from build123d import *

# Parameters (mm, degrees)
SKETCH1_R           = 34.925
BOSS_EXTRUDE1_DEPTH = 146.05
BOSS_EXTRUDE2_DEPTH = 3.175
LPATTERN1_COUNT     = 2
LPATTERN1_PITCH     = 149.225
SKETCH4_R           = 22.225
BOSS_EXTRUDE3_DEPTH = 25.4
SKETCH5_W           = 63.5
SKETCH5_H           = 63.5
BOSS_EXTRUDE4_DEPTH = 50.8
SKETCH6_R           = 9.525
BOSS_EXTRUDE5_DEPTH = 76.2


with BuildPart() as part:
    # Sketch1 → Boss-Extrude1 (new body)
    with BuildSketch(Plane.XY):
        Circle(SKETCH1_R)
    extrude(amount=BOSS_EXTRUDE1_DEPTH)

    # Sketch2 → Boss-Extrude2 (add)
    with BuildSketch(Plane.XY.offset(146.05)):
        Polygon((0, 0), (-38.1, -38.1), (38.1, -38.1), align=None)
    boss_extrude2 = extrude(amount=BOSS_EXTRUDE2_DEPTH)

    # LPattern1: Boss-Extrude2 ×2
    with Locations(*[(0, 0, -i * LPATTERN1_PITCH) for i in range(1, LPATTERN1_COUNT)]):
        add(boss_extrude2)

    # Sketch4 → Boss-Extrude3 (add)
    with BuildSketch(Plane.XY.offset(146.05)):
        with Locations(Location((0, 0, 0), (0, 0, 225))):
            Circle(SKETCH4_R)
    extrude(amount=BOSS_EXTRUDE3_DEPTH)

    # Sketch5 → Boss-Extrude4 (add)
    with BuildSketch(Plane(origin=(0, 33.02, 0), x_dir=(1, 0, 0), z_dir=(0, 1, 0))):
        with Locations((0, -127)):
            Rectangle(SKETCH5_W, SKETCH5_H)
    extrude(amount=BOSS_EXTRUDE4_DEPTH)

    # Sketch6 → Boss-Extrude5 (add)
    with BuildSketch(Plane(origin=(0, 0, 95.25), x_dir=(-1, 0, 0), z_dir=(0, 0, -1))):
        with Locations(Location((0, 74.295, 0), (0, 0, 90))):
            Circle(SKETCH6_R)
    extrude(amount=BOSS_EXTRUDE5_DEPTH)


solid = part.part
Input: part model. Units: mm. Frame: model coordinates. A direction names the side the tool comes from. Round coordinates to 2 decimals unless told otherwise and drop trailing zeros. Loops run counter-clockwise (first coordinate to the right, second up) from the corner with the lowest first, then second, coordinate; pieces in that order, holes last. Notation, with made-up numbers: M 15,11.5 L 57,11.5 A23 cw 57,39.5 Z; hole C 51,19 d9. An arc over 180 degrees is marked long. Answer as CSV lines item,"result". Start each with the question number.
(1) Line query: line 1 (Y direction, x = 0, z = 117) (3 decimals); line 2 (X direction, y = 34, z = 151.5); line 3 (X direction, y = -1.5, z = 60.5). Output: solid intervals per line, ascending. Write a range as [from, to].
(2) First-contact query: pin 1 (1.5 mm diameter, centred on x = 26, y = -22.5, fed in from -Z); pin 2 (15 mm diameter, centred on x = -11, y = 47.5, fed in from +Z); pin 3 (2 mm diameter, centred on x = -24, z = 67.5, fed in from -Y). Flat tips, straight axial feed; report the tip coordinate or a pass-through.
(3) Section D-D, the plane z = 102. Output: boundary loops of the cut face in (x, y) (3 decimals).
(4) Section C-C, the plane z = 45.5. Output: boundary loops of the cut face in (x, y) (3 decimals), plus the area to 3 significant figures.
(5) Section A-A, the plane x = 28. Output: boundary loops of the cut face in (y, z) (3 decimals).
(6) Reachability of faces 5 (the flat face through (31.75, 58, 127)), 6 (the flat face through (0, 74, 19.05)), 7 (the flat face through (27, -27, 148)) from +Z, -Z, +X, -X, +Y, -Y: full face, straight path, thin tool, end or side. Return the list, or none.
(7) Section B-B, the plane y = 49. Output: boundary loops of the cut face in (x, z).
(8) Draft query along Z for faces 1 (the flat face through (-1, -36, 146.05)), 2 (the flat face through (0, 58, 95.25)), 3 (the flat face through (-1, -36, 0)), 4 (the flat face through (19, -19, -2)). Return one class per face: released by +Z, released by -Z, zero draft, split by the parting line, or undercut.
Values found:
1,line 1,"y = [-34.925, 83.82]"
1,line 2,"x = [-31.75, 31.75]"
1,line 3,"x = [-34.89, 34.89]"
2,pin 1,"stops at z = 0"
2,pin 2,"stops at z = 158.75"
2,pin 3,"stops at y = -26.28"
3,outline,"M -31.75,33.02 L -11.377,33.02 A34.925 ccw long 11.377,33.02 L 31.75,33.02 L 31.75,83.82 L -31.75,83.82 Z"
4,outline,"C 0,0 d69.85; C 0,74.295 d19.05"
4,area,"4,120 mm²"
5,outline,"M -38.1,-3.175 L -28,-3.175 L -28,0 L -38.1,0 Z; M -38.1,146.05 L -28,146.05 L -28,149.225 L -38.1,149.225 Z; M -20.875,0 L 20.875,0 L 20.875,146.05 L -20.875,146.05 Z; M 33.02,95.25 L 83.82,95.25 L 83.82,158.75 L 33.02,158.75 Z"
6,face 5,"+Z, -Z, +X, +Y"
6,face 6,"-Z, +X, -X, +Y"
6,face 7,"+Z, +X"
7,outline,"M -31.75,95.25 L 31.75,95.25 L 31.75,158.75 L -31.75,158.75 Z"
8,face 1,"undercut"
8,face 2,"released by -Z"
8,face 3,"undercut"
8,face 4,"zero draft"
